CAD build for the part. Positions are in the model's coordinates, mm. A direction names the side the tool comes from. Coordinates: 2 decimals unless noted, no trailing zeros. Loops run counter-clockwise (first coordinate to the right, second up) from the corner with the lowest first, then second, coordinate; pieces in that order, holes last. Notation, with made-up numbers: (-35, 23) - (-18, 23) arc R18 ccw to (-18, 55) - close; hole circle Ø10 at (79, 18). An arc over 180 degrees is marked (long way). Put each result on its own line as item: value.
Autodesk Inventor part; units mm, degrees
ref_plane "작업 평면3" through (-23.2, 0, 0) normal (1, 0, 0) x (0, 1, 0)
ref_plane "XZ Plane" through (0, 0, 0) normal (0, 1, 0) x (-1, 0, 0)
ref_plane "XY Plane" through (0, 0, 0) normal (0, 0, 1) x (1, 0, 0)
ref_plane "작업 평면10" through (-23.2, 0, 152.9) normal (0, 0, 1) x (1, 0, 0)
sketch "스케치8" plane through (-23.2, 0, 152.9) normal (0, 0, 1) x (1, 0, 0)
  line L0 (17.25, -20.2) -> (-17.25, -20.2)
  line L1 (-17.25, -20.2) -> (-17.25, 20.2)
  line L2 (-17.25, 20.2) -> (17.25, 20.2)
  line L3 (17.25, 20.2) -> (17.25, -20.2)
  circle A0 centre (0, 0) radius 2
  line L4 (-17.25, -20.2) -> (-12.65, -20.2)
  line L5 (-12.65, 20.2) -> (-17.25, 20.2)
  line L6 (-17.25, 20.2) -> (-17.25, -20.2)
  line L7 (17.25, -20.2) -> (12.65, -20.2)
  line L8 (12.65, -20.2) -> (12.65, 20.2)
  line L9 (12.65, 20.2) -> (17.25, 20.2)
  line L10 (17.25, 20.2) -> (17.25, -20.2)
  line L11 (17.25, 20.2) -> (20.85, 20.2)
  line L12 (20.85, 20.2) -> (20.85, -20.2)
  line L13 (20.85, -20.2) -> (17.25, -20.2)
  line L14 (17.25, -20.2) -> (17.25, 20.2)
  line L15 (-17.25, 20.2) -> (-12.65, 20.2)
  line L16 (-12.65, 20.2) -> (-12.65, -20.2)
  line L17 (-12.65, -20.2) -> (-17.25, -20.2)
  line L18 (-17.25, -20.2) -> (-17.25, 20.2)
  line L19 (-17.25, 20.2) -> (-20.85, 20.2)
  line L20 (-20.85, 20.2) -> (-20.85, -20.2)
  line L21 (-17.25, -20.2) -> (-17.25, 20.2)
  line L22 (20.85, 14.5) -> (17.25, 14.5)
  line L23 (17.25, 14.5) -> (17.25, -14.5)
  line L24 (17.25, -14.5) -> (20.85, -14.5)
  line L25 (20.85, -14.5) -> (20.85, 14.5)
  line L26 (0, -20.2) -> (0, 20.2) construction
  line L27 (-17.25, 20.2) -> (-17.25, -20.2)
  circle A1 centre (0, 0) radius 2
  line L28 (-17.25, -20.2) -> (-12.65, -20.2)
  line L29 (-12.65, -20.2) -> (-12.65, 20.2)
  line L30 (-12.65, 20.2) -> (-17.25, 20.2)
  line L31 (-17.25, 20.2) -> (-17.25, -20.2)
  line L32 (-17.25, 20.2) -> (-20.85, 20.2)
  line L33 (-20.85, 20.2) -> (-20.85, -20.2)
  line L34 (-17.25, -20.2) -> (-17.25, 20.2)
  line L35 (-20.85, 14.5) -> (-17.25, 14.5)
  line L36 (-17.25, 14.5) -> (-17.25, -14.5)
  line L37 (-17.25, -14.5) -> (-20.85, -14.5)
  line L38 (-20.85, -14.5) -> (-20.85, 14.5)
  line L39 (-20.85, 20.2) -> (20.85, 20.2)
  line L40 (20.85, 20.2) -> (20.85, 23.2)
  line L41 (20.85, 23.2) -> (-20.85, 23.2)
  line L42 (-20.85, 23.2) -> (-20.85, 20.2)
  line L43 (-17.25, -20.2) -> (-20.85, -20.2)
  line L44 (-20.85, -20.2) -> (20.85, -20.2)
  line L45 (20.85, -20.2) -> (20.85, -23.2)
  line L46 (20.85, -23.2) -> (-20.85, -23.2)
  line L47 (-20.85, -23.2) -> (-20.85, -20.2)
  point P0 (23.2, 0)
  point P1 (-17.25, 0)
  point P2 (20.85, 0)
  point P3 (-23.2, 0)
  point P4 (-20.85, 0)
  point P5 (17.25, 14.5)
  point P6 (20.85, -14.5)
  point P7 (17.25, -14.5)
  point P8 (-17.25, -14.5)
  point P9 (-20.85, -14.5)
  point P10 (-20.85, 14.5)
  point P11 (-17.25, 14.5)
  point P12 (-17.25, 20.2)
  point P13 (20.85, 20.2)
  point P14 (-17.25, 14.5)
  point P15 (-17.25, -14.5)
  point P16 (-20.85, -14.5)
  dimension "d27" = 34.5
  dimension "d30" = 4.6
  dimension "d33" = 29
  dimension "d34" = 40.4
  dimension "d48" = 3
  dimension "d53" = 3
extrude "돌출7" add sketch "스케치8" along normal blind 3 contours L0 L8 L2 L3 | L3 L24 L12 L13 | L0 L16 L2 L8 | L3 L22 L12 L24 | L0 L1 L2 L16 | L3 L11 L12 L22 | L43 L20 L37 L1 | L37 L20 L35 L1 | L1 L35 L20 L19
extrude "돌출8" add sketch "스케치8" along normal blind 61 contours L13 L45 L46 L47 L43 L0 | L3 L24 L12 L13 | L2 L19 L42 L41 L40 L11 | L3 L11 L12 L22 | L43 L20 L37 L1 | L1 L35 L20 L19
ref_plane "작업 평면3" through (-23.2, 0, 0) normal (1, 0, 0) x (0, 1, 0)
sketch "스케치10" plane through (-23.2, 0, 155.9) normal (0, 0, 1) x (1, 0, 0)
  line L0 (-17.25, -14.5) -> (-17.25, -20.2)
  line L1 (-17.25, -20.2) -> (17.25, -20.2)
  line L2 (17.25, -20.2) -> (17.25, -14.5)
  line L3 (17.25, -14.5) -> (20.85, -14.5)
  line L4 (20.85, -14.5) -> (20.85, 14.5)
  line L5 (20.85, 14.5) -> (17.25, 14.5)
  line L6 (17.25, 14.5) -> (17.25, 20.2)
  line L7 (17.25, 20.2) -> (-17.25, 20.2)
  circle A0 centre (0, 0) radius 2
  line L8 (-20.85, -14.75) -> (-17.25, -14.75)
  line L9 (-17.25, -14.75) -> (-17.25, 14.75)
  line L10 (-17.25, 14.75) -> (-20.85, 14.75)
  line L11 (-20.85, 14.75) -> (-20.85, -14.75)
  line L12 (20.85, -14.5) -> (17.25, -14.5)
  line L13 (17.25, -14.5) -> (17.25, 14.5)
  line L14 (17.25, 14.5) -> (20.85, 14.5)
  line L15 (20.85, 14.5) -> (20.85, -14.5)
  line L16 (-17.25, 20.2) -> (-17.25, 14.5)
  line L17 (-17.25, 14.5) -> (-20.85, 14.5)
  line L18 (-20.85, 14.5) -> (-20.85, -14.5)
  line L19 (-20.85, -14.5) -> (-17.25, -14.5)
  point P0 (23.2, 0)
extrude "돌출10" add sketch "스케치10" along normal blind 5.5 contours L19 L11 L17 L9 | L0 L8 L11 L19 | L17 L11 L10 L9 | L13 L5 L4 L3
sketch "스케치11" plane through (-23.2, 0, 155.9) normal (0, 0, 1) x (1, 0, 0)
  circle A0 centre (0, 0) radius 5
  point P0 (23.2, 0)
  dimension "d54" = 10
extrude "돌출11" cut sketch "스케치11" against normal blind 5.5
properties part number "ARM_1 SKETCH"
Q1. Wall check: L1, parallel to Y at x = -23.2, z = 153.85; L2, parallel to Y at x = -29, z = 187; L3, parallel to Z at x = -35, y = -5. Give the ranges that are in metal, low to high. Write a range as from..to.
Determined:
L1: -23.2..-5, 5..23.2
L2: -23.2..-20.2, 20.2..23.2
L3: 152.9..155.9
Q2. Tool access for faces 4 (the flat face through (-23.5, 5.5, 152.9)), 5 (the flat face through (-20, 5, 155.9)), 6 (the flat face through (-4, -14.5, 187)): list every direction of +Z, -Z, +X, -X, +Y, -Y with a clear straight run to the whole face (end or side of a thin tool).
Determined:
face 4: -Z, +X, -X, +Y, -Y
face 5: +Z
face 6: +Z, +X, -X
Q3. Slice it at C-C, the plane z = 185.5. Give the cut face in (x, y), then the cut area to 3 significant figures.
Determined:
outline: (-44.05, -23.2) - (-2.35, -23.2) - (-2.35, -14.5) - (-5.95, -14.5) - (-5.95, -20.2) - (-40.45, -20.2) - (-40.45, -14.5) - (-44.05, -14.5) - close; (-44.05, 14.5) - (-40.45, 14.5) - (-40.45, 20.2) - (-5.95, 20.2) - (-5.95, 14.5) - (-2.35, 14.5) - (-2.35, 23.2) - (-44.05, 23.2) - close
area: 332 mm2
Q4. Slice it at B-B, the plane y = 0. Give the cut face in (x, z).
Determined:
outline: (-44.05, 152.9) - (-28.2, 152.9) - (-28.2, 155.9) - (-40.45, 155.9) - (-40.45, 161.4) - (-44.05, 161.4) - close; (-18.2, 152.9) - (-2.35, 152.9) - (-2.35, 161.4) - (-5.95, 161.4) - (-5.95, 155.9) - (-18.2, 155.9) - close
Q5. Slice it at D-D, the plane y = -19.5. Give the cut face in (x, z), then the cut area to 3 significant figures.
Determined:
outline: (-44.05, 152.9) - (-2.35, 152.9) - (-2.35, 213.9) - (-5.95, 213.9) - (-5.95, 155.9) - (-40.45, 155.9) - (-40.45, 213.9) - (-44.05, 213.9) - close
area: 543 mm2
Q6. Slice it at A-A, the plane x = -23.2. Give the cut face in (y, z), then the cut area to 3 significant figures.
Determined:
outline: (-23.2, 152.9) - (-5, 152.9) - (-5, 155.9) - (-20.2, 155.9) - (-20.2, 213.9) - (-23.2, 213.9) - close; (5, 152.9) - (23.2, 152.9) - (23.2, 213.9) - (20.2, 213.9) - (20.2, 155.9) - (5, 155.9) - close
area: 457 mm2
Q7. Pin check, flat tips, straight feed: pin 1 Ø20 at (y, z) = (-5.5, 189.5) entering from +X; pin 2 Ø11.5 at (x, y) = (-23.2, 0) entering from +Z; pin 3 Ø4 at (x, y) = (-43, 3) entering from +Z. Stop position of each tip, or through.
Determined:
pin 1: x = -2.35
pin 2: z = 155.9
pin 3: z = 161.4
Q8. Mould opens along X. For faces 1 (the flat face through (-4, 14.5, 187)), 2 (the flat face through (-44.05, -16, 183)), 3 (the flat face through (-5.95, 15, 178)) say: +X half, -X half, draft (parallel to the pull), parting line (faces both ways), or undercut.
Determined:
face 1: draft
face 2: -X half
face 3: undercut
